Job drawing, mm, ordinate dimensions from the low corner. One solid piece. Give positions to 0.01 mm unless a question says otherwise; leave off trailing zeros. Loops run counter-clockwise (first coordinate to the right, second up) from the corner with the lowest first, then second, coordinate; pieces in that order, holes last.
Item 1: Saw through at D-D on z = 9.2. Give the cut face in (x, y).
Item 2: Saw through at A-A on z = 16.25. Give the cut face in (x, y).
Item 3: Saw through at C-C on y = 2.2. Give the cut face in (x, z).
Item 4: Saw through at B-B on x = 80. Give the cut face in (y, z), plus the area to 3 significant figures.
Item 5: Probe probe 1 along X at (y, z) = (0.7, 9.2); probe 2 along Z at (x, y) = (80, 1.4); probe 3 along X at (y, z) = (0.7, 13.75). List the from-to ranges inside material, lowest first.
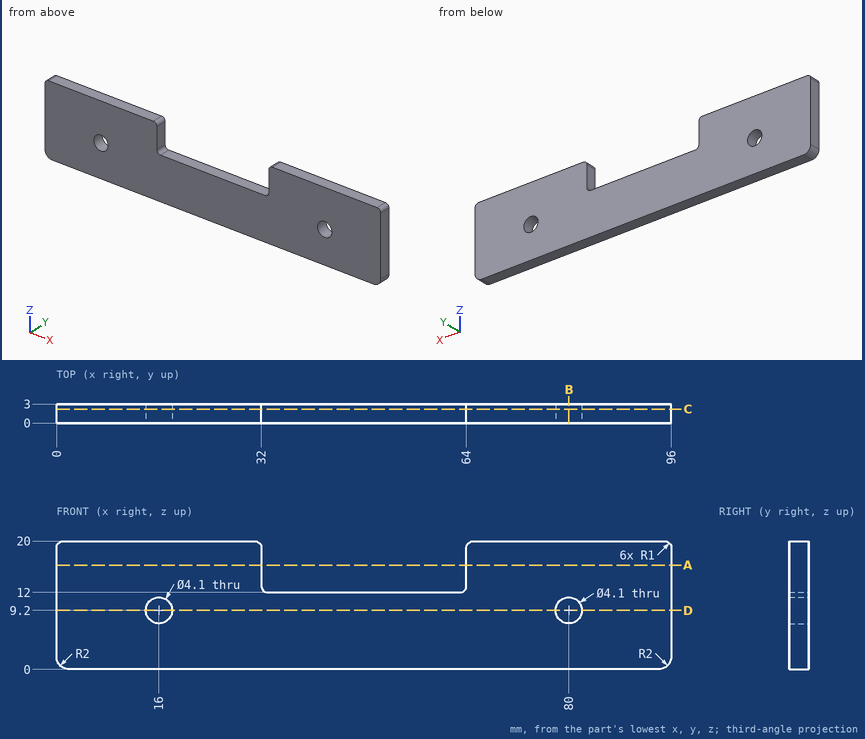
Results below:
1. outline: (0, 0) - (13.95, 0) - (13.95, 3) - (0, 3) - close; (18.05, 0) - (77.95, 0) - (77.95, 3) - (18.05, 3) - close; (82.05, 0) - (96, 0) - (96, 3) - (82.05, 3) - close
2. outline: (0, 0) - (32, 0) - (32, 3) - (0, 3) - close; (64, 0) - (96, 0) - (96, 3) - (64, 3) - close
3. outline: (0, 2) arc R2 ccw to (2, 0) - (94, 0) arc R2 ccw to (96, 2) - (96, 19) arc R1 ccw to (95, 20) - (65, 20) arc R1 ccw to (64, 19) - (64, 13) arc R1 cw to (63, 12) - (33, 12) arc R1 cw to (32, 13) - (32, 19) arc R1 ccw to (31, 20) - (1, 20) arc R1 ccw to (0, 19) - close; hole circle Ø4.1 at (16, 9.2); hole circle Ø4.1 at (80, 9.2)
4. outline: (0, 0) - (3, 0) - (3, 7.15) - (0, 7.15) - close; (0, 11.25) - (3, 11.25) - (3, 20) - (0, 20) - close
4. area: 47.7 mm2
5. probe 1: x = 0 to 13.95, 18.05 to 77.95, 82.05 to 96
5. probe 2: z = 0 to 7.15, 11.25 to 20
5. probe 3: x = 0 to 32, 64 to 96
